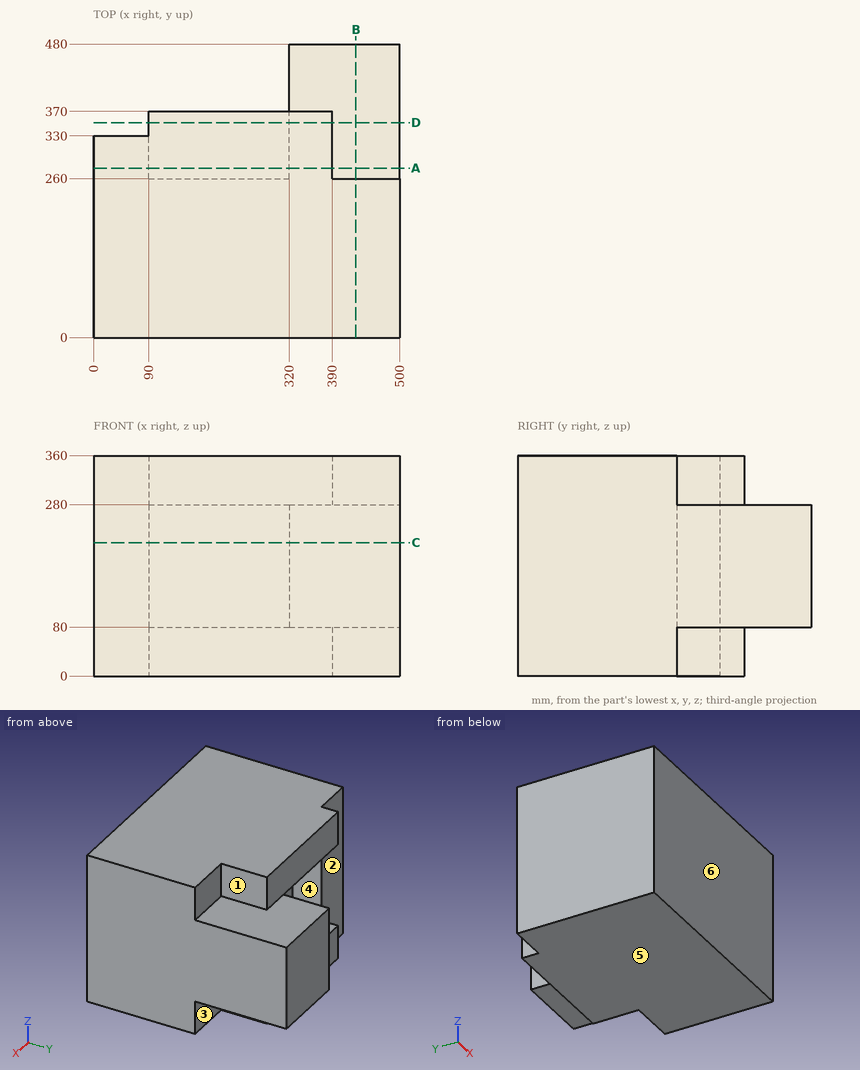
Check sheet for the drawn part. Datum: minimum x, y, z corner. Units: mm. A direction names the side the tool comes from. Give positions to 0.01 mm unless a question says otherwise; leave off trailing zeros. Write each loop counter-clockwise with the first axis right and the second up, starting at its lowest first coordinate (ties: lowest second). Pieces come first, ordered by that corner, then holes.
(1) Cross-section at A-A (y = 277). Enter the section's corners in (x, z).
(2) Gauge pin test, flat ends, axial feed: pin 1 (12 mm diameter, centred on x = 295, y = 203.5, fed in from -Z); pin 2 (24 mm diameter, centred on x = 419.5, z = 43, fed in from +Y). Record the tip position at first contact, or that the pin passes through.
(3) Material ranges on line 1 (X direction, y = 310.5, z = 93); line 2 (X direction, y = 432.5, z = 209); line 3 (Y direction, x = 115.5, z = 177.5), recorded low to high.
(4) Cross-section at C-C (z = 218). Enter the section's corners in (x, y), plus the area to 3 significant figures.
(5) Mould release check, pull along Z, two halves, no side actions. Record for the marked faces 4, 5 and 6: +Z half, -Z half, draft (parallel to the pull), parting line (faces both ways), or undercut.
(6) Access from +Z, -Z, +X, -X, +Y, -Y to the whole of each face (thin tool, end or side, straight path). Record for the marked faces 1, 2 and 3.
(7) Cross-section at D-D (y = 351.5). Enter the section's corners in (x, z).
(8) Cross-section at B-B (x = 428.5). Enter the section's corners in (y, z).
Worked out:
1. outline: (0, 0) - (390, 0) - (390, 80) - (500, 80) - (500, 280) - (390, 280) - (390, 360) - (0, 360) - close; hole (90, 80) - (320, 80) - (320, 280) - (90, 280) - close
2. pin 1: stops at z = 0
2. pin 2: stops at y = 260
3. line 1: x = 0 to 90, 320 to 500
3. line 2: x = 320 to 500
3. line 3: y = 0 to 260
4. outline: (0, 0) - (500, 0) - (500, 480) - (320, 480) - (320, 260) - (90, 260) - (90, 330) - (0, 330) - close
4. area: 176,000 mm2
5. face 4: undercut
5. face 5: -Z half
5. face 6: draft
6. face 1: +Z, +X, +Y
6. face 2: +Z, -Z, -X, +Y
6. face 3: -Z, +X, +Y
7. outline: (90, 0) - (390, 0) - (390, 80) - (500, 80) - (500, 280) - (390, 280) - (390, 360) - (90, 360) - (90, 280) - (320, 280) - (320, 80) - (90, 80) - close
8. outline: (0, 0) - (260, 0) - (260, 80) - (480, 80) - (480, 280) - (260, 280) - (260, 360) - (0, 360) - close
